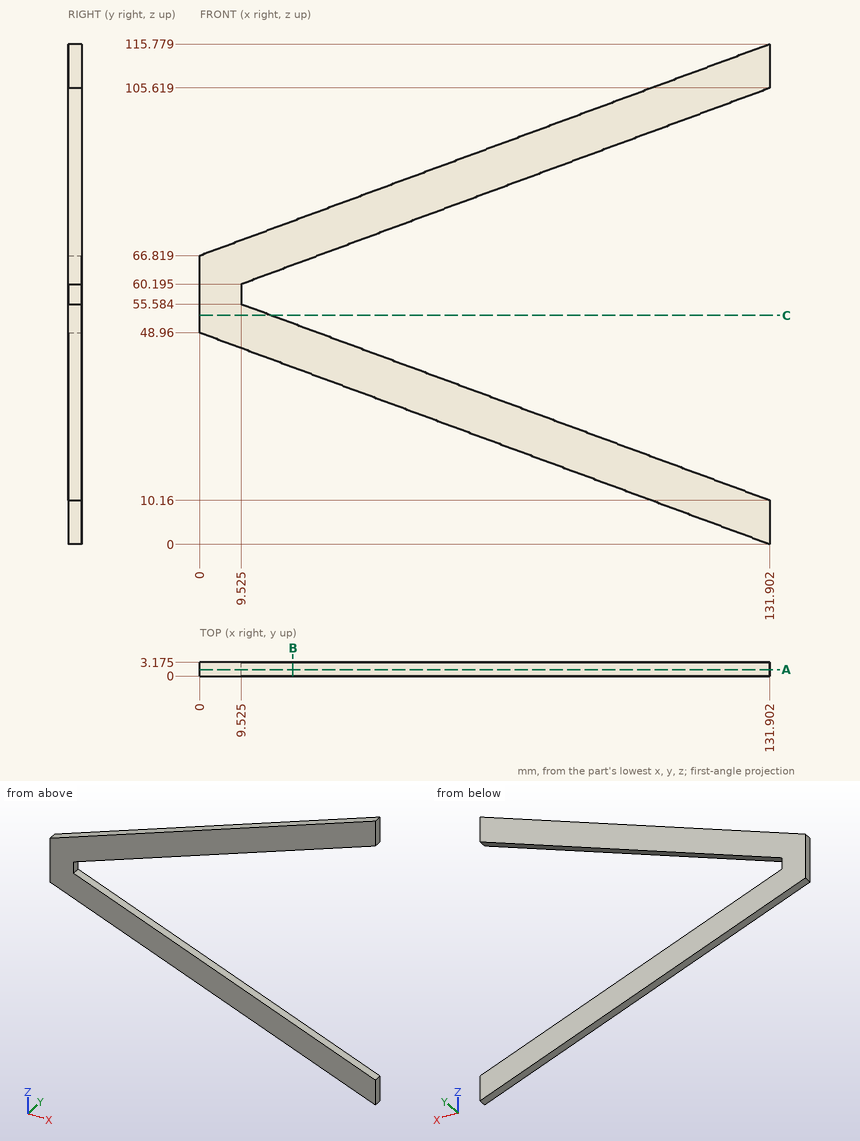
Part print with two shaded views. Sizes in mm from the minimum x, y, z corner. Round coordinates to 2 decimals unless told otherwise and drop trailing zeros. Loops run counter-clockwise (first coordinate to the right, second up) from the corner with the lowest first, then second, coordinate; pieces in that order, holes last. Notation, with made-up numbers: (42.5, 72.25) - (68.5, 72.25) arc R14 ccw to (68.5, 99.25) - close; hole circle Ø1 at (69.25, 56). An arc over 180 degrees is marked (long way). Put each result on its own line as item: value.
1. Slice it at B-B on x = 21.5. List the corners of the cut face in (y, z) (1 decimal).
Geometry check:
outline: (0, 41) - (3.2, 41) - (3.2, 51.1) - (0, 51.1) - close; (0, 64.6) - (3.2, 64.6) - (3.2, 74.8) - (0, 74.8) - close
2. Wall check: line 1 (Z direction, x = 51.5, y = 0.4) (1 decimal); line 2 (Z direction, x = 79.5, y = 2). Give the ranges that are in metal, low to high.
Geometry check:
line 1: 29.8 to 40, 75.8 to 85.9
line 2: 19.45 to 29.61, 86.17 to 96.33
3. Pin check, flat tips, straight feed: P1, Ø1.5, axis at x = 45, y = 1, coming from the -Z side; P2, Ø1, axis at y = 1, z = 57.5, coming from the +X side (3 decimals). Stop position of each tip, or through.
Geometry check:
P1: z = 31.98
P2: x = 9.525
4. Slice it at C-C on z = 53. List the corners of the cut face in (x, y) (1 decimal).
Geometry check:
outline: (0, 0) - (16.5, 0) - (16.5, 3.2) - (0, 3.2) - close
5. Slice it at A-A on y = 1.5. List the corners of the cut face in (x, z) (1 decimal), and give its area (3 significant figures).
Geometry check:
outline: (0, 49) - (131.9, 0) - (131.9, 10.2) - (9.5, 55.6) - (9.5, 60.2) - (131.9, 105.6) - (131.9, 115.8) - (0, 66.8) - close
area: 2,690 mm²
